Model file for the job. Use its own axes, mm. A direction names the side the tool comes from. Round coordinates to 2 decimals unless told otherwise and drop trailing zeros. Order: outer loops, then holes, each group sorted by start corner. A loop starts at its lowest first (then second) coordinate and runs counter-clockwise, first axis right, second up. Notation, with made-up numbers: (27.25, 47.5) - (62.25, 47.5) arc R10 cw to (62.25, 55.5) - close; hole circle Ø4 at (-39.75, 25). An arc over 180 degrees is marked (long way). Write item = value, one per line.
```python
from build123d import *

# Parameters (mm, degrees)
F0_R     = 12.7
F1_DEPTH = 50.8
F2_W     = 5.08
F2_H     = 9.525
F4_SIZE  = 3.81
F6_D     = 5.1054


with BuildPart() as f1:
    # F0 (on Top) → F1 (new body)
    with BuildSketch(Plane.XY):
        Circle(F0_R)
    extrude(amount=F1_DEPTH)

    # F2 (on Right) → F3 (revolve, cut)
    with BuildSketch(Plane.YZ):
        with Locations((-10.16, 30.1625)):
            Rectangle(F2_W, F2_H)
    revolve(axis=Axis((0, 0, 34.6962809563), (0, 0, 1)), mode=Mode.SUBTRACT)

    # F4
    f4_edges = [f1.edges().sort_by_distance(p)[0] for p in [
        (-12.7, 0, 34.925),
        (-12.7, 0, 25.4),
    ]]
    chamfer(f4_edges, length=F4_SIZE)

    # F6 (through all)
    with Locations(Plane(origin=(0, 0, 0), x_dir=(1, 0, 0), z_dir=(0, 0, -1))):
        with Locations((0, 0)):
            Hole(F6_D / 2)


solid = f1.part
```
1) Wall check: line 1 along Z through (x, y) = (-6.25, -6.25) (3 decimals); line 2 along Y through (x, z) = (0, 12); line 3 along Z through (x, y) = (8.5, -4.25). Give the ranges that are in metal, low to high.
Conclusion:
line_1 = 0 to 25.4, 34.925 to 50.8
line_2 = -12.7 to -2.55, 2.55 to 12.7
line_3 = 0 to 24.79, 35.54 to 50.8
2) Mould opens along Y. For faces 1 (the face through (-2.435, -0.767, 25.756)), 2 (the face through (-2.75, -12.4, 10.64)), 3 (the face through (4, -7, 25.4)) say: +Y half, -Y half, draft (parallel to the pull), parting line (faces both ways), or undercut.
Conclusion:
face_1 = undercut
face_2 = parting line
face_3 = draft
3) Cut at A-A (y = 0). Write the cut outline in (x, z) (3 decimals).
Conclusion:
outline = (-12.7, 0) - (-2.553, 0) - (-2.553, 50.8) - (-12.7, 50.8) - (-12.7, 38.735) - (-8.89, 34.925) - (-7.62, 34.925) - (-7.62, 25.4) - (-8.89, 25.4) - (-12.7, 21.59) - close; (2.553, 0) - (12.7, 0) - (12.7, 21.59) - (8.89, 25.4) - (7.62, 25.4) - (7.62, 34.925) - (8.89, 34.925) - (12.7, 38.735) - (12.7, 50.8) - (2.553, 50.8) - close
4) Flat gauge pins, fed straight in: pin 1 Ø5 at (x, z) = (7, 17.5) entering from +Y; pin 2 Ø1 at (x, z) = (-5, 12) entering from -Y; pin 3 Ø3 at (y, z) = (-10, 30) entering from +X; pin 4 Ø8 at (x, z) = (-7, 31.5) entering from +Y. Where does each tip first touch, or does it go through?
Conclusion:
pin_1 = 11.88
pin_2 = -11.88
pin_3 = through
pin_4 = 7.4
5) 3-axis set-ups, long thin cutter, end or side, ignore diameter. For faces 4 (the face through (4, -7, 34.925)), 5 (the face through (3, 0, 0)): which of +Z, -Z, +X, -X, +Y, -Y reach the whole face in a straight line?
Conclusion:
face_4 = none
face_5 = -Z, +X, -X, +Y, -Y
6) Cut at C-C (z = 23). Write the cut outline in (x, y), and give its area (3 significant figures).
Conclusion:
outline = circle Ø22.58 at (0, 0); hole circle Ø5.11 at (0, 0)
area = 380 mm^2
